Input: part model. Units: mm. Frame: model coordinates. Face numbers are marked on the shaded views. Round coordinates to 2 decimals unless told otherwise and drop trailing zeros. Loops run counter-clockwise (first coordinate to the right, second up) from the corner with the lowest first, then second, coordinate; pieces in that order, holes last. Notation, with made-up numbers: (78, -22) - (115, -22) arc R15 ccw to (115, 2) - close; hole circle Ø4 at (14.5, 1). An arc over 180 degrees is marked (long way). One line per question, with ' | ' between items. Start each with the question number.
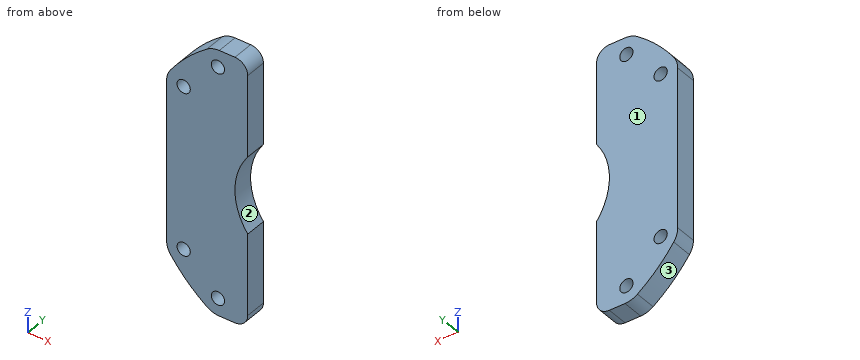
from build123d import *

# Parameters (mm, degrees)
EXTRUDE_1_DEPTH     = 5
SKETCH_2_R          = 15
CUT_EXTRUDE_1_DEPTH = 10
SKETCH_3_R          = 1.55
CUT_EXTRUDE_2_DEPTH = 10
SKETCH_7_W          = 49.108203812
SKETCH_7_H          = 84.922292299
CUT_EXTRUDE_4_DEPTH = 10
FILLET_1_R          = 3
FILLET_2_R          = 5


with BuildPart() as part:
    # 草图1 → 凸台-拉伸1 (new body)
    with BuildSketch(Plane(origin=(0, 0, 0), x_dir=(1, 0, 0), z_dir=(0, 1, 0))):
        with BuildLine():
            Line((-20.199009877, 31), (20.199009877, 31))
            ThreePointArc((20.199009877, 31), (26.162950904, 26.162950904), (31, 20.199009877))
            Line((31, 20.199009877), (31, -20.199009877))
            ThreePointArc((31, -20.199009877), (26.162950904, -26.162950904), (20.199009877, -31))
            Line((20.199009877, -31), (-20.199009877, -31))
            ThreePointArc((-20.199009877, -31), (-26.162950904, -26.162950904), (-31, -20.199009877))
            Line((-31, -20.199009877), (-31, 20.199009877))
            ThreePointArc((-31, 20.199009877), (-26.162950904, 26.162950904), (-20.199009877, 31))
        make_face()
    extrude(amount=EXTRUDE_1_DEPTH)

    # 草图2 → 切除-拉伸1 (cut)
    with BuildSketch(Plane(origin=(0, 5, 0), x_dir=(1, 0, 0), z_dir=(0, 1, 0))):
        with Locations(Location((0, 0, 0), (0, 0, 270))):
            Circle(SKETCH_2_R)
    extrude(amount=-CUT_EXTRUDE_1_DEPTH, mode=Mode.SUBTRACT)

    # 草图3 → 切除-拉伸2 (cut)
    with BuildSketch(Plane(origin=(0, 5, 0), x_dir=(1, 0, 0), z_dir=(0, 1, 0))):
        with Locations(Location((-26.998940675, 18.975173317, 0), (0, 0, 270))):
            Circle(SKETCH_3_R)
        with Locations(Location((-18.975173317, 26.998940675, 0), (0, 0, 270))):
            Circle(SKETCH_3_R)
        with Locations(Location((26.998940675, 18.975173317, 0), (0, 0, 270))):
            Circle(SKETCH_3_R)
        with Locations(Location((18.975173317, 26.998940675, 0), (0, 0, 270))):
            Circle(SKETCH_3_R)
        with Locations(Location((26.998940675, -18.975173317, 0), (0, 0, 270))):
            Circle(SKETCH_3_R)
        with Locations(Location((18.975173317, -26.998940675, 0), (0, 0, 270))):
            Circle(SKETCH_3_R)
        with Locations(Location((-26.998940675, -18.975173317, 0), (0, 0, 270))):
            Circle(SKETCH_3_R)
        with Locations(Location((-18.975173317, -26.998940675, 0), (0, 0, 270))):
            Circle(SKETCH_3_R)
    extrude(amount=-CUT_EXTRUDE_2_DEPTH, mode=Mode.SUBTRACT)

    # 草图7 → 切除-拉伸4 (cut)
    with BuildSketch(Plane(origin=(0, 5, 0), x_dir=(1, 0, 0), z_dir=(0, 1, 0))):
        with Locations((12.554101906, 6.469881358)):
            Rectangle(SKETCH_7_W, SKETCH_7_H)
    extrude(amount=-CUT_EXTRUDE_4_DEPTH, mode=Mode.SUBTRACT)

    # 圆角1
    fillet_1_edges = [part.edges().sort_by_distance(p)[0] for p in [
        (-12, 2.5, 31),
        (-12, 2.5, -31),
    ]]
    fillet(fillet_1_edges, radius=FILLET_1_R)

    # 圆角2
    fillet_2_edges = [part.edges().sort_by_distance(p)[0] for p in [
        (-20.199009877, 2.5, -31),
        (-20.199009877, 2.5, 31),
        (-31, 2.5, 20.199009877),
        (-31, 2.5, -20.199009877),
    ]]
    fillet(fillet_2_edges, radius=FILLET_2_R)


solid = part.part
(1) Section B-B, the plane x = -19.5. Output: boundary loops of the cut face in (y, z), plus the area to 3 significant figures.
(2) Section D-D, the plane x = -23. Output: boundary loops of the cut face in (y, z), plus the area to 3 significant figures.
(3) Pull-direction query (Z, two-part tool) for the marked faces 1, 2 and 3; classes: released by +Z, released by -Z, zero draft, split by the parting line, or undercut.
(4) Section C-C, the plane y = 2.9. Output: boundary loops of the cut face in (x, z), plus the area to 3 significant figures.
(5) Line query: line 1 along Z through (x, y) = (-20, 2.85); line 2 along X through (y, z) = (4.05, 0.5); line 3 along Z through (x, y) = (-13.25, 4.8). Output: solid intervals per line, ascending. Write a range as from..to.
(6) Section A-A, the plane z = 27. Output: boundary loops of the cut face in (x, y).
Derived:
1) outline: (0, -30.93) - (5, -30.93) - (5, -28.46) - (0, -28.46) - close; (0, -25.54) - (5, -25.54) - (5, 25.54) - (0, 25.54) - close; (0, 28.46) - (5, 28.46) - (5, 30.93) - (0, 30.93) - close | area: 280 mm²
2) outline: (0, -28.98) - (5, -28.98) - (5, 28.98) - (0, 28.98) - close | area: 290 mm²
3) face 1: zero draft | face 2: undercut | face 3: released by -Z
4) outline: (-31, -18.65) arc R5 ccw to (-30.06, -21.57) arc R37 ccw to (-21.57, -30.06) arc R5 ccw to (-18.65, -31) - (-15, -31) arc R3 ccw to (-12, -28) - (-12, -9) arc R15 cw to (-12, 9) - (-12, 28) arc R3 ccw to (-15, 31) - (-18.65, 31) arc R5 ccw to (-21.57, 30.06) arc R37 ccw to (-30.06, 21.57) arc R5 ccw to (-31, 18.65) - close; hole circle Ø3.1 at (-27, -18.98); hole circle Ø3.1 at (-27, 18.98); hole circle Ø3.1 at (-18.98, -27); hole circle Ø3.1 at (-18.98, 27) | area: 1,010 mm²
5) line 1: z = -30.82..-28.16, -25.84..25.84, 28.16..30.82 | line 2: x = -31..-14.99 | line 3: z = -30.44..-7.03, 7.03..30.44
6) outline: (-25.3, 0) - (-20.53, 0) - (-20.53, 5) - (-25.3, 5) - close; (-17.43, 0) - (-12, 0) - (-12, 5) - (-17.43, 5) - close
